Source: CAD feature listing. Evaluate the final solid. Frame: model axes, mm. Face numbers are marked on the shaded views. A direction names the side the tool comes from. Coordinates: 2 decimals unless noted, no trailing zeros. Order: outer loops, then holes, each group sorted by start corner. A loop starts at its lowest first (then second) coordinate and runs counter-clockwise, first axis right, second up. Notation, with made-up numbers: (1, 84) - (19, 84) arc R19 ccw to (19, 100) - close; hole circle Ø8 at (64.5, 4.5). An arc over 180 degrees is marked (long way). One line per question, with ' | ' between items. Start each with the question number.
(1) Access query for the marked faces 1, 2 and 3. Directions: +Z, -Z, +X, -X, +Y, -Y. A direction counts if a zero-diameter tool reaches every point of the face in a straight line with its end or side. Return the directions, or none.
(2) Line query: line 1 along Z through (x, y) = (-67, 0.45) (3 decimals); line 2 along X through (y, z) = (0.5, -88) (3 decimals); line 3 along X through (y, z) = (3, -34.5). Output: solid intervals per line, ascending.
(3) Section A-A (z = -88). Return the cut outline in (x, y) (1 decimal).
(4) Section C-C (x = -24.5). Return the cut outline in (y, z), then the cut area to 3 significant figures.
(5) Contact query for flat-ended pins moving along their axis: P1, Ø6, axis at x = -71, z = -77, coming from the +Y side; P2, Ø1.2, axis at x = -73.5, z = 9.5, coming from the -Y side; P3, Ø2, axis at y = 28.5, z = -16.5, coming from the -X side; P4, Ø1, axis at x = -73.5, z = -114, coming from the +Y side. Output: stop coordinate, or through.
(6) Section D-D (z = -63.5). Return the cut outline in (x, y), then the cut area to 3 significant figures.
(7) Section B-B (x = -67). Count the separate pieces of the cut face and the enclosed holes in it, then the cut area to 3 significant figures.
Autodesk Inventor part; units mm, degrees
ref_plane "YZ Plane" through (0, 0, 0) normal (1, 0, 0) x (0, 1, 0)
ref_plane "XZ Plane" through (0, 0, 0) normal (0, 1, 0) x (-1, 0, 0)
ref_plane "XY Plane" through (0, 0, 0) normal (0, 0, 1) x (1, 0, 0)
sketch "Sketch3" plane through (0, 0, 0) normal (0, 1, 0) x (-1, 0, 0)
  line L0 (0, 0) -> (70, 0)
  line L1 (70, 0) -> (70, -70)
  line L2 (70, -70) -> (70, -94)
  line L3 (70, -94) -> (64, -94)
  line L4 (64, -94) -> (64, -70)
  line L5 (64, -3) -> (0, -3)
  line L6 (0, -3) -> (0, 0)
  line L7 (64, -70) -> (67, -70)
  line L8 (67, -70) -> (67, -3)
  line L9 (67, -3) -> (64, -3)
  circle A0 centre (67, -82) radius 2.125
  circle A1 centre (67, -76) radius 2.125
  circle A2 centre (67, -88) radius 2.125
  dimension "d26" = 70
  dimension "d27" = 70
  dimension "d29" = 6
  dimension "d55" = 4.25
  dimension "d56" = 4.25
  dimension "d57" = 4.25
  dimension "d59" = 6
  dimension "d60" = 6
  dimension "d61" = 6
extrude "Extrusion2" add sketch "Sketch3" along normal blind 27 contours L0 L1 L2 L3 L4 L7 L8 L9 L5 L6 | A0 | A1 | A2
sketch "Sketch4" plane through (0, 27, 0) normal (0, 1, 0) x (1, 0, 0)
  line L0 (-70, 0) -> (0, 0)
  line L1 (0, 0) -> (0, 3)
  line L2 (-70, 0) -> (0, 0)
  line L3 (0, 0) -> (0, 3)
  line L4 (0, 3) -> (-70, 3)
  line L5 (-70, 3) -> (-70, 0)
extrude "Extrusion3" add sketch "Sketch4" along normal blind 20
sketch "Sketch5" plane through (-70, 0, -94) normal (-1, 0, 0) x (0, 0, 1)
  line L0 (-0.1204, 1.5) -> (23.8796, 1.5)
  line L1 (23.8796, 1.5) -> (23.8796, 25.5)
  line L2 (23.8796, 25.5) -> (-0.1204, 25.5)
  line L3 (-0.1204, 25.5) -> (-0.1204, 1.5)
  line L4 (94, 0) -> (0, 0)
  dimension "d36" = 24
  dimension "d37" = 24
  dimension "d38" = 1.5
extrude "Extrusion4" cut sketch "Sketch5" against normal blind 10
sketch "Sketch9" plane through (0, 0, -3) normal (0, 0, -1) x (-1, 0, 0)
  line L0 (7, 7) -> (60, 7)
  line L1 (60, 7) -> (60, 39)
  line L2 (60, 39) -> (7, 39)
  line L3 (7, 39) -> (7, 7)
  line L4 (0, 0) -> (0, 47)
  line L5 (67, 0) -> (0, 0)
  dimension "d45" = 53
  dimension "d46" = 32
  dimension "d47" = 7
  dimension "d48" = 7
extrude "Extrusion5" cut sketch "Sketch9" against normal blind 10
sketch "Sketch10" plane through (-70, 0, 0) normal (0, 0, 1) x (1, 0, 0)
  line L0 (10, 39) -> (10, 7)
  line L1 (63, 7) -> (63, 39)
  line L2 (63, 26.6385) -> (63, 18.6385)
  line L3 (10, 18.6385) -> (10, 26.6385)
  line L4 (63, 39) -> (10, 39)
  line L5 (10, 7) -> (63, 7)
  line L6 (31.6097, 39) -> (39.6097, 39)
  line L7 (39.6097, 39) -> (39.6097, 7)
  line L8 (39.6097, 7) -> (31.6097, 7)
  line L9 (31.6097, 7) -> (31.6097, 18.6385)
  line L10 (31.6097, 26.6385) -> (31.6097, 39)
  line L11 (10, 26.6385) -> (31.6097, 26.6385)
  line L12 (39.6097, 26.6385) -> (63, 26.6385)
  line L13 (63, 18.6385) -> (39.6097, 18.6385)
  line L14 (31.6097, 18.6385) -> (10, 18.6385)
  point P0 (70, 0)
  dimension "d51" = 8
  dimension "d52" = 8
extrude "Extrusion6" add sketch "Sketch10" against normal blind 3 contours L11 L10 L4 L7 L5 L9 L14 L0 | L12 L1 L13 L7
sketch "Sketch11" plane through (0, 0, 0) normal (0, -1, 0) x (1, 0, 0)
  point P0 (0, 0)
sketch "Sketch12" plane through (0, 0, 0) normal (0, -1, 0) x (1, 0, 0)
  circle A0 centre (-67, -82) radius 2.125
  circle A1 centre (-67, -76) radius 2.125
  circle A2 centre (-67, -88) radius 2.125
  line L0 (-64, -70) -> (-67, -70)
  point P0 (0, 0)
  dimension "d62" = 4.25
  dimension "d63" = 4.25
  dimension "d64" = 4.25
  dimension "d65" = 6
  dimension "d66" = 6
  dimension "d67" = 6
hole "Hole2" at (-67, 0, -88) at (-67, 0, -82) at (-67, 0, -76) direction (0, 1, 0) diameter 4.25 end through all
sketch "Sketch15" plane through (-67, 0, -3) normal (1, 0, 0) x (0, 0, -1)
  line L0 (67, 0) -> (67, 27)
  line L1 (67, 0) -> (0, 0)
  line L2 (67, 0) -> (0, 0)
  line L3 (0, 0) -> (0, 27)
  line L4 (0, 0) -> (0, 27)
  line L5 (0, 27) -> (67, 27)
  line L6 (67.1204, 25.5) -> (67.1204, 1.5)
  line L7 (67.1204, 25.5) -> (67.1204, 1.5)
  line L8 (67.1204, 1.5) -> (67, 0)
  line L9 (67, 27) -> (67, 0)
  point P0 (-3, 0)
extrude "Extrusion7" add sketch "Sketch15" along normal blind 3
sketch "Sketch18" plane through (-64, 0, -3) normal (1, 0, 0) x (0, 0, -1)
  line L0 (0, 0) -> (0, 27)
  line L1 (0, 27) -> (0, 0)
  line L2 (91, 0) -> (0, 0)
  line L3 (0, 0) -> (91, 0)
  line L4 (91, 0) -> (91, 1.5)
  line L5 (91, 0) -> (91, 1.5)
  line L6 (67.1204, 1.5) -> (67.1204, 25.5)
  line L7 (91, 1.5) -> (67.1204, 1.5)
  line L8 (67.1204, 25.5) -> (67.1204, 1.5)
  line L9 (67.1204, 1.5) -> (67.1204, 25.5)
  line L10 (67.1204, 25.5) -> (91, 25.5)
  line L11 (67.1204, 25.5) -> (91, 25.5)
  line L12 (91, 27) -> (0, 27)
  line L13 (91, 25.5) -> (91, 27)
  line L14 (91, 27) -> (0, 27)
  point P0 (-3, 0)
extrude "Extrusion8" add sketch "Sketch18" along normal blind 1
sketch "Sketch19" plane through (-70, 0, -94) normal (-1, 0, 0) x (0, 0, 1)
  line L0 (94, 47) -> (94, 0)
  line L1 (91, 0) -> (0, 0)
  line L2 (94, 0) -> (0, 0)
  line L3 (0, 0) -> (0, 1.5)
  line L4 (0, 0) -> (0, 1.5)
  line L5 (23.8796, 25.5) -> (23.8796, 1.5)
  line L6 (0, 1.5) -> (23.8796, 1.5)
  line L7 (23.8796, 1.5) -> (23.8796, 25.5)
  line L8 (23.8796, 25.5) -> (0, 25.5)
  line L9 (23.8796, 25.5) -> (0, 25.5)
  line L10 (0, 27) -> (91, 27)
  line L11 (0, 25.5) -> (0, 27)
  line L12 (0, 27) -> (91, 27)
  line L13 (91, 27) -> (91, 47)
  line L14 (91, 27) -> (91, 47)
  line L15 (91, 47) -> (94, 47)
  line L16 (91, 47) -> (94, 47)
extrude "Extrusion9" add sketch "Sketch19" along normal blind 1
sketch "Sketch20" plane through (-71, 0, -94) normal (-1, 0, 0) x (0, 0, 1)
  line L0 (94, 26.6385) -> (94, 39)
  line L1 (94, 26.6385) -> (114.5, 26.6385)
  line L2 (114.5, 26.6385) -> (114.5, 18.6385)
  line L3 (94, 18.6385) -> (94, 7)
  line L4 (114.5, 18.6385) -> (94, 18.6385)
  line L5 (94, 18.6385) -> (0, 18.6385)
  line L6 (0, 18.6385) -> (-20.5, 18.6385)
  line L7 (-20.5, 18.6385) -> (-20.5, 26.6385)
  line L8 (-20.5, 26.6385) -> (94, 26.6385)
  point P0 (94, 0)
  dimension "d81" = 20.5
  dimension "d82" = 94
  dimension "d83" = 20.5
  dimension "d84" = 180
extrude "Extrusion10" add sketch "Sketch20" along normal blind 2
sketch "Sketch21" plane through (-71, 0, -94) normal (-1, 0, 0) x (0, 0, 1)
  line L0 (94, 18.6385) -> (94, 7)
  line L1 (94, 0) -> (94, 18.6385)
  line L2 (94, 18.6385) -> (23.8796, 18.6385)
  line L3 (94, 18.6385) -> (23.8796, 18.6385)
  line L4 (23.8796, 1.5) -> (23.8796, 25.5)
  line L5 (23.8796, 18.6385) -> (23.8796, 1.5)
  line L6 (91, 0) -> (0, 0)
  line L7 (23.8796, 1.5) -> (0, 1.5)
  line L8 (23.8796, 1.5) -> (0, 1.5)
  line L9 (0, 1.5) -> (0, 0)
  line L10 (0, 1.5) -> (0, 0)
  line L11 (0, 0) -> (94, 0)
extrude "Extrusion11" add sketch "Sketch21" along normal blind 2
sketch "Sketch22" plane through (-71, 0, -94) normal (-1, 0, 0) x (0, 0, 1)
  line L0 (91, 27) -> (0, 27)
  line L1 (0, 27) -> (0, 26.6385)
  line L2 (0, 27) -> (0, 26.6385)
  line L3 (0, 25.5) -> (0, 27)
  line L4 (94, 26.6385) -> (94, 47)
  line L5 (0, 26.6385) -> (94, 26.6385)
  line L6 (94, 26.6385) -> (94, 47)
  line L7 (94, 47) -> (91, 47)
  line L8 (94, 47) -> (91, 47)
  line L9 (91, 47) -> (91, 27)
  line L10 (91, 47) -> (91, 27)
  line L11 (91, 27) -> (0, 27)
  point P0 (94, 0)
extrude "Extrusion12" add sketch "Sketch22" along normal blind 2
sketch "Sketch23" plane through (-73, 0, -94) normal (-1, 0, 0) x (0, 0, 1)
  line L0 (94, 0) -> (94, 47)
  line L1 (94, 18.6385) -> (94, 26.6385)
  line L2 (94, 0) -> (94, 18.6385)
  line L3 (114.5, 18.6385) -> (114.5, 26.6385)
  line L4 (94, 18.6385) -> (114.5, 18.6385)
  line L5 (114.5, 18.6385) -> (114.5, 26.6385)
  line L6 (114.5, 26.6385) -> (94, 26.6385)
  line L7 (94, 26.6385) -> (94, 47)
  line L8 (94, 47) -> (91, 47)
  line L9 (94, 47) -> (91, 47)
  line L10 (0, 27) -> (91, 27)
  line L11 (91, 47) -> (91, 27)
  line L12 (91, 26.6385) -> (91, 39)
  line L13 (91, 27) -> (0, 27)
  line L14 (0, 26.6385) -> (-20.5, 26.6385)
  line L15 (0, 27) -> (0, 26.6385)
  line L16 (0, 25.5) -> (0, 27)
  line L17 (0, 26.6385) -> (-20.5, 26.6385)
  line L18 (-20.5, 26.6385) -> (-20.5, 18.6385)
  line L19 (-20.5, 26.6385) -> (-20.5, 18.6385)
  line L20 (-20.5, 18.6385) -> (23.8796, 18.6385)
  line L21 (-20.5, 18.6385) -> (23.8796, 18.6385)
  line L22 (23.8796, 18.6385) -> (23.8796, 1.5)
  line L23 (23.8796, 18.6385) -> (23.8796, 1.5)
  line L24 (0, 1.5) -> (0, 0)
  line L25 (23.8796, 1.5) -> (0, 1.5)
  line L26 (0, 1.5) -> (0, 0)
  line L27 (0, 0) -> (94, 0)
  line L28 (0, 0) -> (94, 0)
extrude "Extrusion13" add sketch "Sketch23" along normal blind 2
sketch "Sketch24" plane through (-75, 0, -94) normal (-1, 0, 0) x (0, 0, 1)
  line L0 (-17.5, 26.6385) -> (-17.5, 25.1385)
  line L1 (-17.5, 25.1385) -> (-18.5, 25.1385)
  line L2 (-18.5, 25.1385) -> (-18.5, 26.6385)
  line L3 (-17.5, 26.6385) -> (-17.5, 25.1385)
  line L4 (-17.5, 26.6385) -> (-18.5, 26.6385)
  line L5 (-20.5, 26.6385) -> (0, 26.6385)
  line L6 (-20.5, 18.6385) -> (-20.5, 26.6385)
  line L7 (-20.5, 22.6385) -> (-27.0892, 22.6385)
  line L8 (-17.5, 18.6385) -> (-17.5, 20.1385)
  line L9 (-17.5, 20.1385) -> (-18.5, 20.1385)
  line L10 (-18.5, 20.1385) -> (-18.5, 18.6385)
  line L11 (-17.5, 18.6385) -> (-18.5, 18.6385)
  line L12 (91, 0) -> (0, 0)
  line L13 (45.5, 0) -> (45.5, 18.6385)
  line L14 (108.5, 26.6385) -> (108.5, 25.1385)
  line L15 (108.5, 25.1385) -> (109.5, 25.1385)
  line L16 (109.5, 25.1385) -> (109.5, 26.6385)
  line L17 (108.5, 18.6385) -> (108.5, 20.1385)
  line L18 (108.5, 20.1385) -> (109.5, 20.1385)
  line L19 (109.5, 20.1385) -> (109.5, 18.6385)
  line L20 (108.5, 18.6385) -> (109.5, 18.6385)
  line L21 (108.5, 26.6385) -> (109.5, 26.6385)
  line L22 (94, 26.6385) -> (114.5, 26.6385)
  point P0 (94, 0)
  dimension "d93" = 17.5
  dimension "d94" = 1.5
  dimension "d95" = 1
extrude "Extrusion14" cut sketch "Sketch24" against normal through all
properties part number "GrapperRight"
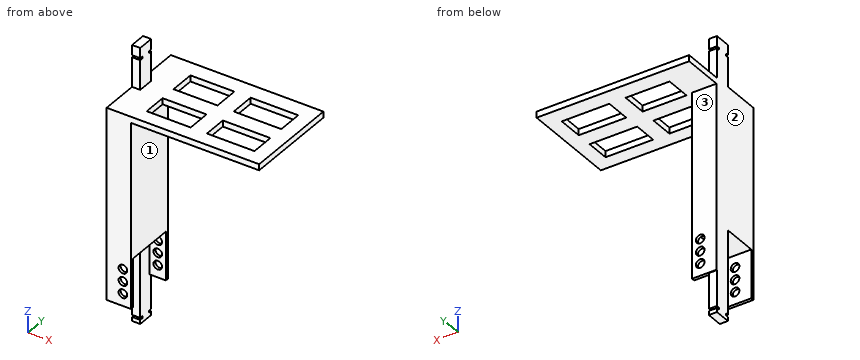
Response values:
1) face 1: -Z, +X, +Y, -Y | face 2: +Z, -Z, -X, +Y, -Y | face 3: -Z, +X, -X, +Y
2) line 1: z = -94 to -90.125, -85.875 to -84.125, -79.875 to -78.125, -73.875 to 0 | line 2: x = -75 to -69.125, -64.875 to -63 | line 3: x = -75 to -63
3) outline: (-75, 0) - (-69.1, 0) - (-69.1, 1.5) - (-75, 1.5) - close; (-75, 18.6) - (-71, 18.6) - (-71, 25.5) - (-69.1, 25.5) - (-69.1, 27) - (-75, 27) - close; (-64.9, 0) - (-63, 0) - (-63, 1.5) - (-64.9, 1.5) - close; (-64.9, 25.5) - (-63, 25.5) - (-63, 27) - (-64.9, 27) - close
4) outline: (0, -3) - (7, -3) - (7, 0) - (0, 0) - close; (18.64, -3) - (26.64, -3) - (26.64, 0) - (18.64, 0) - close; (39, -3) - (47, -3) - (47, 0) - (39, 0) - close | area: 69.0 mm²
5) P1: stops at y = 27 | P2: stops at y = 18.64 | P3: passes through | P4: stops at y = 26.64
6) outline: (-75, 0) - (-63, 0) - (-63, 27) - (-75, 27) - close | area: 324 mm²
7) separate pieces: 7 | enclosed holes: 0 | area: 1,990 mm²
